Design review of the part shown in the three views and the two pictorial views. Dimensions are in mm from the part's minimum x, y and z. A direction names the side the tool comes from. Coordinates: 2 decimals unless noted, no trailing zeros. Loops run counter-clockwise (first coordinate to the right, second up) from the corner with the lowest first, then second, coordinate; pieces in that order, holes last. Notation, with made-up numbers: (-3.5, -36) -> (7.5, -36) arc R8 cw to (7.5, -25) -> close; hole circle Ø7 at (-36, 5.5). An arc over 180 degrees is marked (long way). Answer in a Markdown table with one row per item.
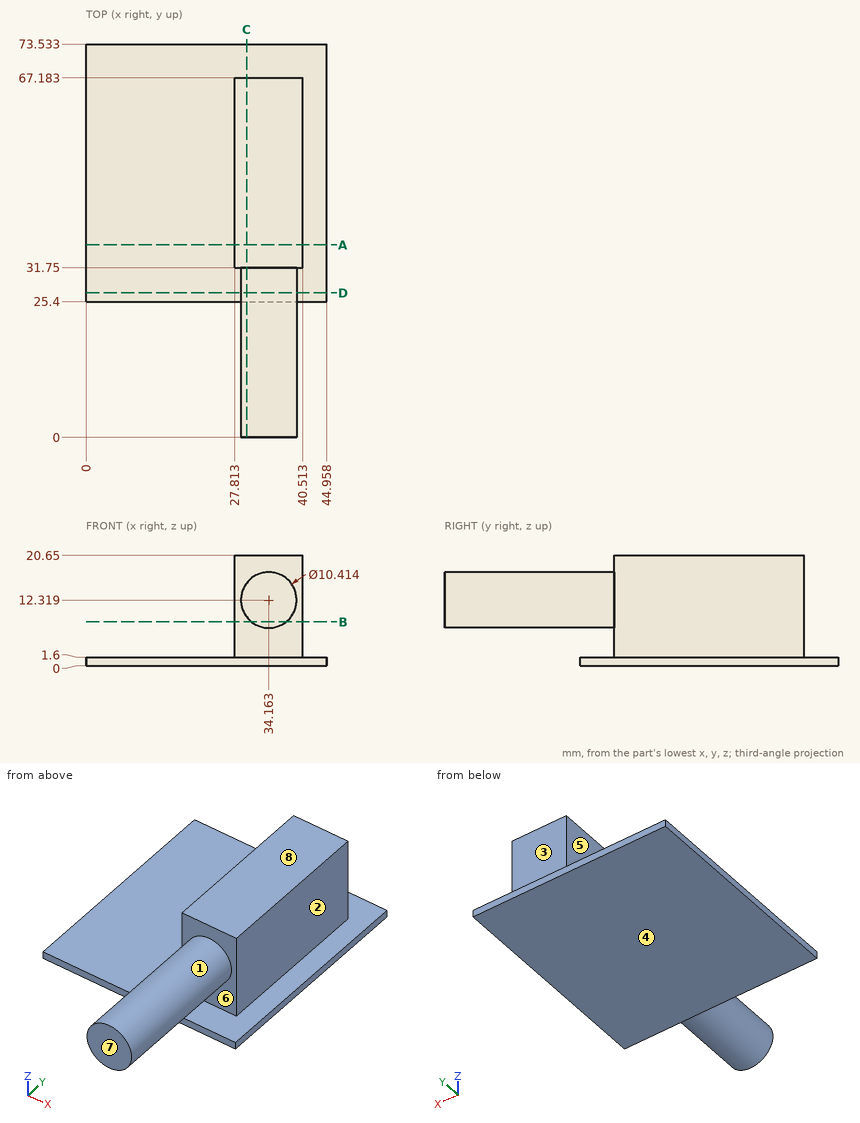
Item 1: Take a section at C-C, the plane x = 30. State the section outline as (y, z) points, and give its area (3 significant figures).
Worked answers:
| item | result |
|---|---|
| outline | (0, 9.19) -> (31.75, 9.19) -> (31.75, 1.6) -> (25.4, 1.6) -> (25.4, 0) -> (73.53, 0) -> (73.53, 1.6) -> (67.18, 1.6) -> (67.18, 20.65) -> (31.75, 20.65) -> (31.75, 15.45) -> (0, 15.45) -> close |
| area | 951 mm² |
Item 2: For L1, parallel to Y at x = 39.5, z = 17; L2, parallel to Z at x = 23, y = 52.5; L3, parallel to X at y = 64.5, z = 4.75, list the stretches that pass through material, from the lowest coordinate up.
Worked answers:
| item | result |
|---|---|
| L1 | 31.75 to 67.18 |
| L2 | 0 to 1.6 |
| L3 | 27.81 to 40.51 |
Item 3: Take a section at A-A, the plane y = 36. State the section outline as (x, z) points.
Worked answers:
| item | result |
|---|---|
| outline | (0, 0) -> (44.96, 0) -> (44.96, 1.6) -> (40.51, 1.6) -> (40.51, 20.65) -> (27.81, 20.65) -> (27.81, 1.6) -> (0, 1.6) -> close |
Item 4: Take a section at D-D, the plane y = 27. State the section outline as (x, z) points, and give its area (3 significant figures).
Worked answers:
| item | result |
|---|---|
| outline | (0, 0) -> (44.96, 0) -> (44.96, 1.6) -> (0, 1.6) -> close; circle Ø10.41 at (34.16, 12.32) |
| area | 157 mm² |
Item 5: Insertion check: pin 1 (12 mm diameter, centred on x = 18.5, z = 7, fed in from -Y); pin 2 (5 mm diameter, centred on x = 27, z = 12, fed in from +Y); pin 3 (2 mm diameter, centred on y = 29.5, z = 13.5, fed in from -X). Each pin has a flat end and moves straight along its axis. Give the tip position at first contact, or say it passes through.
Worked answers:
| item | result |
|---|---|
| pin 1 | y = 25.4 |
| pin 2 | y = 67.18 |
| pin 3 | x = 28.96 |
Item 6: Take a section at B-B, the plane z = 8.25. State the section outline as (x, y) points.
Worked answers:
| item | result |
|---|---|
| outline | (27.81, 31.75) -> (30.91, 31.75) -> (30.91, 0) -> (37.41, 0) -> (37.41, 31.75) -> (40.51, 31.75) -> (40.51, 67.18) -> (27.81, 67.18) -> close |
Item 7: For the marked faces 1, 2, 3, 4 and 5, list the 3-axis set-ups (+Z, -Z, +X, -X, +Y, -Y) from which the entire face can be reached by the end or side of a thin tool; tool diameter is ignored.
Worked answers:
| item | result |
|---|---|
| face 1 | -Y |
| face 2 | +Z, +X, +Y, -Y |
| face 3 | +Z, +X, -X, +Y |
| face 4 | -Z, +X, -X, +Y, -Y |
| face 5 | +Z, -X, +Y, -Y |
Item 8: The part is to be moulded in two halves that separate along Z. For the marked faces 6, 7 and 8, say which applies: +Z half, -Z half, draft (parallel to the pull), parting line (faces both ways), or undercut.
Worked answers:
| item | result |
|---|---|
| face 6 | undercut |
| face 7 | draft |
| face 8 | +Z half |
